CAD build for the part. Positions are in the model's coordinates, mm. Face numbers are marked on the shaded views. A direction names the side the tool comes from. Coordinates: 2 decimals unless noted, no trailing zeros. Loops run counter-clockwise (first coordinate to the right, second up) from the corner with the lowest first, then second, coordinate; pieces in that order, holes last. Notation, with made-up numbers: M 78,83 L 108,83 A22 ccw 108,111 Z; hole C -21,77.25 d11. An arc over 180 degrees is marked long. Answer as a JSON object with one key per item and string values. Group by question number.
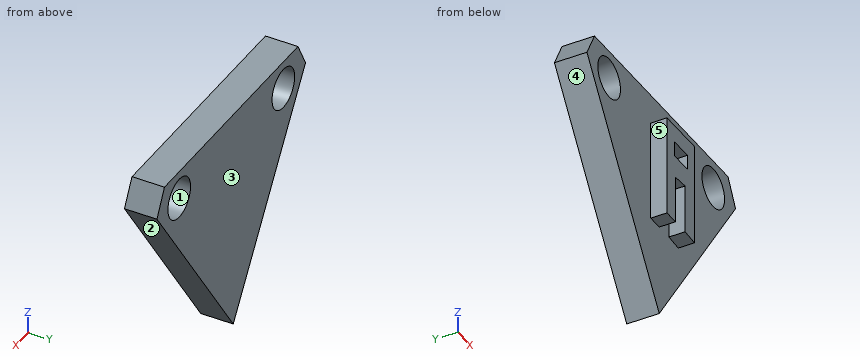
```python
from build123d import *

# Parameters (mm, degrees)
F1_DEPTH = 5.08
F2_R     = 3.175
F3_DEPTH = 5.081
F4_W     = 3.626744
F4_H     = 2.346717
F5_DEPTH = 2.54


with BuildPart() as f1:
    # F0 (on Front) → F1 (new body)
    with BuildSketch(Plane.XZ):
        Polygon((-27.176633, 47.891983), (-29.307042, 43.846673), (-8.993444, 12.680604), (12.433227, 43.568405), (10.31143, 47.61824), align=None)
    extrude(amount=F1_DEPTH)

    # F2 (on face) → F3 (cut, through all)
    with BuildSketch(Plane.XZ.offset(5.08)):
        with Locations((6.172628, 43.203343)):
            Circle(F2_R)
        with Locations((-23.074293, 43.416909)):
            Circle(F2_R)
    extrude(amount=-F3_DEPTH, mode=Mode.SUBTRACT)

    # F4 (on face) → F5 (join)
    with BuildSketch(Plane.XZ.offset(5.08)):
        Polygon((-3.665128, 43.108057), (-11.393237, 43.108057), (-11.393237, 27.177891), (-8.993444, 27.177891), (-8.993444, 34.644719), (-6.305161, 34.846445), (-6.305161, 27.177891), (-3.665128, 26.964553), align=None)
        with Locations((-7.447374, 39.231487)):
            Rectangle(F4_W, F4_H, mode=Mode.SUBTRACT)
    extrude(amount=F5_DEPTH)


solid = f1.part
```
Item 1: Slice it at A-A, the plane y = -7. Write the cut outline in (x, z).
Item 2: Drill centre lines: L1, parallel to X at y = -0.5, z = 45.5; L2, parallel to X at y = -2, z = 44.5; L3, parallel to Z at x = -24, y = -3. Where is each one in solid material? Low to high. Write a range as from..to.
Item 3: Pull direction X, two halves, no side cores. Call the marked faces 1, 2 and 3: released by +X, released by -X, zero draft, split by the parting line, or undercut.
Item 4: Slice it at B-B, the plane x = -22.5. Write the cut outline in (y, z), then the cut area to 3 significant figures.
Item 5: Slice it at D-D, the plane x = -8. Write the cut outline in (y, z), then the cut area to 3 significant figures.
Item 6: Tool access for the marked faces 4 and 5: list every direction of +Z, -Z, +X, -X, +Y, -Y with a clear straight run to the whole face (end or side of a thin tool).
Item 7: Slice it at C-C, the plane z = 45.5. Write the cut outline in (x, y).
Item 8: Pin check, flat tips, straight feed: pin 1 (1 mm diameter, centred on y = -2, z = 23.5, fed in from +X); pin 2 (0.8 mm diameter, centred on x = -8, y = -6.5, fed in from +Z); pin 3 (1.3 mm diameter, centred on y = -5.5, z = 31, fed in from +X). Stop position of each tip, or through.
Computed:
{
 "1": {"outline": "M -11.39,27.18 L -8.99,27.18 L -8.99,34.64 L -6.31,34.85 L -6.31,27.18 L -3.67,26.96 L -3.67,43.11 L -11.39,43.11 Z; hole M -9.26,38.06 L -5.63,38.06 L -5.63,40.4 L -9.26,40.4 Z"},
 "2": {"L1": "-28.44..-25.47, -20.68..3.98, 8.36..11.42", "L2": "-28.96..-26.06, -20.09..3.27, 9.07..11.95", "L3": "35.7..40.38, 46.45..47.87"},
 "3": {"face 1": "undercut", "face 2": "released by +X", "face 3": "zero draft"},
 "4": {"outline": "M -5.08,33.4 L 0,33.4 L 0,40.29 L -5.08,40.29 Z; M -5.08,46.54 L 0,46.54 L 0,47.86 L -5.08,47.86 Z", "area": "41.7 mm2"},
 "5": {"outline": "M -7.62,34.72 L -5.08,34.72 L -5.08,14.11 L 0,14.11 L 0,47.75 L -5.08,47.75 L -5.08,43.11 L -7.62,43.11 L -7.62,40.4 L -5.08,40.4 L -5.08,38.06 L -7.62,38.06 Z", "area": "186 mm2"},
 "6": {"face 4": "-Z, -X, +Y, -Y", "face 5": "+Z, -Z, -X, -Y"},
 "7": {"outline": "M -28.44,-5.08 L -25.47,-5.08 L -25.47,0 L -28.44,0 Z; M -20.68,-5.08 L 3.98,-5.08 L 3.98,0 L -20.68,0 Z; M 8.36,-5.08 L 11.42,-5.08 L 11.42,0 L 8.36,0 Z"},
 "8": {"pin 1": "x = -1.14", "pin 2": "z = 43.11", "pin 3": "x = 4.06"}
}
